Verification items for the finished model (mm, model axes). Face numbers are marked on the shaded views. A direction names the side the tool comes from. Round coordinates to 2 decimals unless told otherwise and drop trailing zeros. Write each loop counter-clockwise with the first axis right and the second up, starting at its lowest first coordinate (ties: lowest second). Pieces come first, ordered by that corner, then holes. Notation, with made-up numbers: M 75.25,24 L 103.25,24 A15 cw 103.25,38 Z; hole C 12.5,13.5 d10. An arc over 180 degrees is marked long. Answer in a Markdown table with one row per item. Add a question column.
1. Material ranges on probe 1 along X at (y, z) = (-2.2, -37); probe 2 along X at (y, z) = (-1.25, 43.6); probe 3 along X at (y, z) = (-2.15, -13.6), recorded low to high.
2. Sectioned sample at B-B on z = -13.6. Record the cut outline in (x, y).
3. Sectioned sample at C-C on y = -21. Record the cut outline in (x, z).
4. Sectioned sample at A-A on x = -45. Record the cut outline in (y, z), plus the area to 3 significant figures.
5. Set-up check for the marked faces 1, 2 and 3: record each of +Z, -Z, +X, -X, +Y, -Y from which the full face is reachable in a straight line by a thin tool's end or side.
6. Go/stop test with flat-tipped pins: pin 1 Ø12 at (y, z) = (-24, -36) entering from +X; pin 2 Ø5 at (x, z) = (-44, -8.5) entering from -Y; pin 3 Ø15 at (y, z) = (-38.5, -22) entering from -X. Record where each tip stops, or that it passes through.
7. Sectioned sample at D-D on x = 52.5. Record the cut outline in (y, z), plus the area to 3 significant figures.
```python
from build123d import *

# Parameters (mm, degrees)
SKETCH1_R           = 5
SKETCH1_R_2         = 3
BOSS_EXTRUDE2_DEPTH = 5
BOSS_EXTRUDE3_DEPTH = 5
FILLET1_R           = 20
FILLET2_R           = 5


with BuildPart() as part:
    # Sketch1 → Boss-Extrude2 (new body)
    with BuildSketch(Plane(origin=(0, 0, 0), x_dir=(1, 0, 0), z_dir=(0, 1, 0))):
        with BuildLine():
            Line((60, 2.8), (60, 50))
            Line((60, 50), (-60, 50))
            Line((-60, 50), (-60, 2.8))
            Line((-60, 2.8), (-35, 2.8))
            ThreePointArc((-35, 2.8), (-17.2, -15), (-35, -32.8))
            Line((-35, -32.8), (-60, -32.8))
            Line((-60, -32.8), (-60, -55))
            Line((-60, -55), (60, -55))
            Line((60, -55), (60, -32.8))
            Line((60, -32.8), (35, -32.8))
            ThreePointArc((35, -32.8), (17.2, -15), (35, 2.8))
            Line((35, 2.8), (60, 2.8))
        make_face()
        with Locations(Location((-35, 13.6, 0), (0, 0, 270))):
            Circle(SKETCH1_R, mode=Mode.SUBTRACT)
        with Locations(Location((-35, -43.6, 0), (0, 0, 270))):
            Circle(SKETCH1_R, mode=Mode.SUBTRACT)
        with Locations(Location((35, 13.6, 0), (0, 0, 270))):
            Circle(SKETCH1_R, mode=Mode.SUBTRACT)
        with Locations(Location((35, -43.6, 0), (0, 0, 270))):
            Circle(SKETCH1_R, mode=Mode.SUBTRACT)
        with Locations(Location((-45, 37, 0), (0, 0, 270))):
            Circle(SKETCH1_R_2, mode=Mode.SUBTRACT)
        with Locations(Location((-25, 37, 0), (0, 0, 270))):
            Circle(SKETCH1_R_2, mode=Mode.SUBTRACT)
        with Locations(Location((25, 37, 0), (0, 0, 270))):
            Circle(SKETCH1_R_2, mode=Mode.SUBTRACT)
        with Locations(Location((45, 37, 0), (0, 0, 270))):
            Circle(SKETCH1_R_2, mode=Mode.SUBTRACT)
    extrude(amount=-BOSS_EXTRUDE2_DEPTH)

    # Sketch2 → Boss-Extrude3 (add, symmetric)
    with BuildSketch(Plane(origin=(0, 0, 0), x_dir=(0, 0, -1), z_dir=(1, 0, 0))):
        Polygon((-10, -5), (50, -55), (50, -5), align=None)
    extrude(amount=BOSS_EXTRUDE3_DEPTH, both=True)

    # Fillet1
    fillet1_edges = [part.edges().sort_by_distance(p)[0] for p in [
        (60, -2.5, -2.8),
        (-60, -2.5, -2.8),
    ]]
    fillet(fillet1_edges, radius=FILLET1_R)

    # Fillet2
    fillet2_edges = [part.edges().sort_by_distance(p)[0] for p in [
        (60, -2.5, -50),
        (60, -2.5, 32.8),
        (60, -2.5, 55),
        (-60, -2.5, 55),
        (-60, -2.5, 32.8),
        (-60, -2.5, -50),
    ]]
    fillet(fillet2_edges, radius=FILLET2_R)


solid = part.part
```
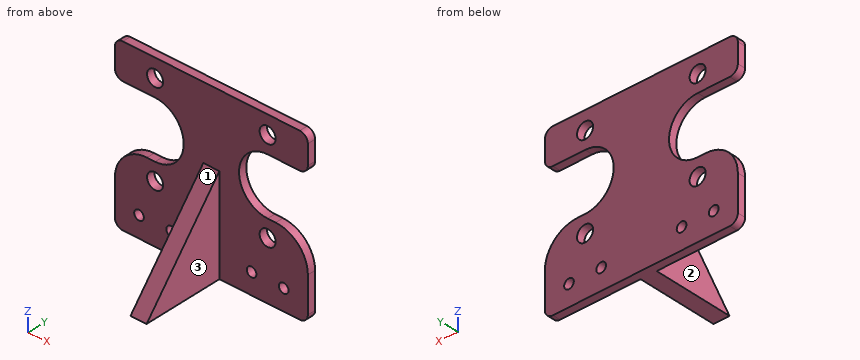
Geometry check:
| question | item | result |
|---|---|---|
| 1 | probe 1 | x = -60 to -48, -42 to -28, -22 to 22, 28 to 42, 48 to 60 |
| 1 | probe 2 | x = -60 to -40, -30 to 30, 40 to 60 |
| 1 | probe 3 | x = -57.76 to -40, -30 to 30, 40 to 57.76 |
| 2 | outline | M -57.76,-5 L -40,-5 L -40,0 L -57.76,0 Z; M -30,-5 L -5,-5 L -5,-24.67 L 5,-24.67 L 5,-5 L 30,-5 L 30,0 L -30,0 Z; M 40,-5 L 57.76,-5 L 57.76,0 L 40,0 Z |
| 3 | outline | M -5,-50 L 5,-50 L 5,-9.2 L -5,-9.2 Z |
| 4 | outline | M -5,-50 L 0,-50 L 0,-40 L -5,-40 Z; M -5,-34 L 0,-34 L 0,-3.44 L -5,-3.44 Z; M -5,32.8 L 0,32.8 L 0,55 L -5,55 Z |
| 4 | area | 314 mm2 |
| 5 | face 1 | +Z, +X, -X, -Y |
| 5 | face 2 | +Z, -Z, -X, -Y |
| 5 | face 3 | +Z, -Z, +X, -Y |
| 6 | pin 1 | stops at x = 5 |
| 6 | pin 2 | stops at y = -5 |
| 6 | pin 3 | stops at x = -5 |
| 7 | outline | M -5,-50 L 0,-50 L 0,-7.19 L -5,-7.19 Z; M -5,32.8 L 0,32.8 L 0,55 L -5,55 Z |
| 7 | area | 325 mm2 |
